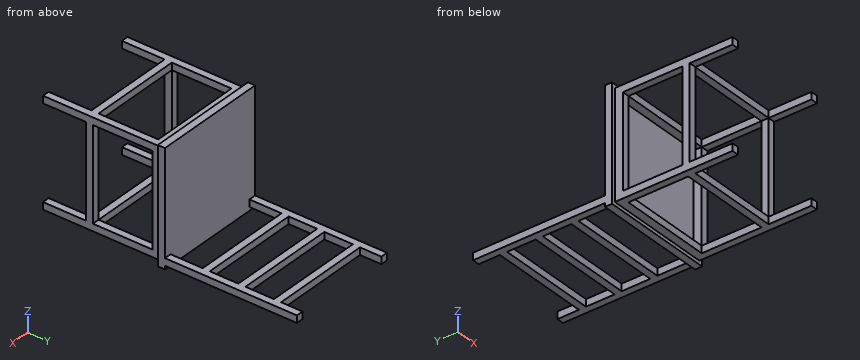
```python
from build123d import *

# Parameters (mm, degrees)
SKETCH1_W            = 406.4
SKETCH1_H            = 406.4
BOSS_EXTRUDE1_DEPTH  = 25.4
SKETCH2_W            = 25.4
SKETCH2_H            = 25.4
SKETCH2_W_2          = 330.2
SKETCH2_H_2          = 330.2
BOSS_EXTRUDE4_DEPTH  = 28.575
SKETCH4_W            = 25.4
SKETCH4_H            = 25.4
BOSS_EXTRUDE5_DEPTH  = 390.525
SKETCH6_W            = 25.4
SKETCH6_H            = 25.4
BOSS_EXTRUDE6_DEPTH  = 355.6
SKETCH8_W            = 25.4
SKETCH8_H            = 25.4
BOSS_EXTRUDE7_DEPTH  = 355.6
SKETCH9_W            = 25.4
SKETCH9_H            = 25.4
BOSS_EXTRUDE8_DEPTH  = 355.6
SKETCH10_W           = 25.4
SKETCH10_H           = 25.4
BOSS_EXTRUDE9_DEPTH  = 355.6
SKETCH11_W           = 25.4
SKETCH11_H           = 25.4
BOSS_EXTRUDE11_DEPTH = 469.9
SKETCH12_W           = 25.4
SKETCH12_H           = 25.4
BOSS_EXTRUDE12_DEPTH = 376.174


with BuildPart() as part:
    # Sketch1 → Boss-Extrude1 (new body)
    with BuildSketch(Plane(origin=(0, 0, 0), x_dir=(1, 0, 0), z_dir=(0, 1, 0))):
        with Locations((203.2, 203.2)):
            Rectangle(SKETCH1_W, SKETCH1_H)
    extrude(amount=BOSS_EXTRUDE1_DEPTH)

    # Sketch2 → Boss-Extrude4 (add)
    with BuildSketch(Plane.XZ):
        with Locations((25.4, -25.4)):
            Rectangle(SKETCH2_W, SKETCH2_H)
        with Locations((203.2, -25.4)):
            Rectangle(SKETCH2_W_2, SKETCH2_H)
        with Locations((25.4, -203.2)):
            Rectangle(SKETCH2_W, SKETCH2_H_2)
        with Locations((203.2, -381)):
            Rectangle(SKETCH2_W_2, SKETCH2_H)
        with Locations((25.4, -381)):
            Rectangle(SKETCH2_W, SKETCH2_H)
        with Locations((381, -381)):
            Rectangle(SKETCH2_W, SKETCH2_H)
        with Locations((381, -203.2)):
            Rectangle(SKETCH2_W, SKETCH2_H_2)
        with Locations((381, -25.4)):
            Rectangle(SKETCH2_W, SKETCH2_H)
    extrude(amount=BOSS_EXTRUDE4_DEPTH)

    # Sketch4 → Boss-Extrude5 (add)
    with BuildSketch(Plane.XZ.offset(28.575)):
        with Locations((25.4, -25.4)):
            Rectangle(SKETCH4_W, SKETCH4_H)
        with Locations((381, -25.4)):
            Rectangle(SKETCH4_W, SKETCH4_H)
        with Locations((381, -381)):
            Rectangle(SKETCH4_W, SKETCH4_H)
        with Locations((25.4, -381)):
            Rectangle(SKETCH4_W, SKETCH4_H)
    extrude(amount=BOSS_EXTRUDE5_DEPTH)

    # Sketch6 → Boss-Extrude6 (add)
    with BuildSketch(Plane(origin=(38.1, 0, 0), x_dir=(0, 0, -1), z_dir=(1, 0, 0))):
        with Locations((25.4, -254)):
            Rectangle(SKETCH6_W, SKETCH6_H)
    extrude(amount=BOSS_EXTRUDE6_DEPTH)

    # Sketch8 → Boss-Extrude7 (add)
    with BuildSketch(Plane(origin=(0, 0, -38.1), x_dir=(-1, 0, 0), z_dir=(0, 0, -1))):
        with Locations((-381, -254)):
            Rectangle(SKETCH8_W, SKETCH8_H)
    extrude(amount=BOSS_EXTRUDE7_DEPTH)

    # Sketch9 → Boss-Extrude8 (add)
    with BuildSketch(Plane.ZY.offset(-368.3)):
        with Locations((-381, -254)):
            Rectangle(SKETCH9_W, SKETCH9_H)
    extrude(amount=BOSS_EXTRUDE8_DEPTH)

    # Sketch10 → Boss-Extrude9 (add)
    with BuildSketch(Plane.XY.offset(-368.3)):
        with Locations((25.4, -254)):
            Rectangle(SKETCH10_W, SKETCH10_H)
    extrude(amount=BOSS_EXTRUDE9_DEPTH)

    # Sketch11 → Boss-Extrude11 (add)
    with BuildSketch(Plane(origin=(0, 25.4, 0), x_dir=(1, 0, 0), z_dir=(0, 1, 0))):
        with Locations((12.7, 381)):
            Rectangle(SKETCH11_W, SKETCH11_H)
        with Locations((393.7, 381)):
            Rectangle(SKETCH11_W, SKETCH11_H)
    extrude(amount=BOSS_EXTRUDE11_DEPTH)

    # Sketch12 → Boss-Extrude12 (add)
    with BuildSketch(Plane.ZY.offset(-381)):
        with Locations((-381, 406.4)):
            Rectangle(SKETCH12_W, SKETCH12_H)
        with Locations((-381, 279.4)):
            Rectangle(SKETCH12_W, SKETCH12_H)
        with Locations((-381, 152.4)):
            Rectangle(SKETCH12_W, SKETCH12_H)
    extrude(amount=BOSS_EXTRUDE12_DEPTH)


solid = part.part
```
Check sheet for the modelled part. Datum: model origin and axes. Units: mm. Give positions to 0.01 mm unless a question says otherwise; leave off trailing zeros. Loops run counter-clockwise (first coordinate to the right, second up) from the corner with the lowest first, then second, coordinate; pieces in that order, holes last. Notation, with made-up numbers: M 10.25,88 L 18.25,88 A17 cw 18.25,94 Z; hole C 0,-23.75 d1. An arc over 180 degrees is marked long. Answer in a Markdown table with one row per item.
1) Cross-section at A-A (x = 265). Count the separate pieces of the cut face and the enclosed holes in it, plus the area to 3 significant figures.
Solutions:
| item | result |
|---|---|
| separate pieces | 6 |
| enclosed holes | 0 |
| area | 15,000 mm^2 |
2) Cross-section at C-C (y = 329). Enter the section's corners in (x, z), plus the area to 3 significant figures.
Solutions:
| item | result |
|---|---|
| outline | M 0,-393.7 L 25.4,-393.7 L 25.4,-368.3 L 0,-368.3 Z; M 381,-393.7 L 406.4,-393.7 L 406.4,-368.3 L 381,-368.3 Z |
| area | 1,290 mm^2 |
3) Thickness scan on line 1 (X direction, y = -252, z = -318); line 2 (Z direction, x = 363.5, y = -1.5); line 3 (Y direction, x = 204, z = -21.5) (3 decimals). Record the ranges inside material, lowest first.
Solutions:
| item | result |
|---|---|
| line 1 | x = 12.7 to 38.1, 368.3 to 393.7 |
| line 2 | z = -393.7 to -368.3, -38.1 to -12.7 |
| line 3 | y = -266.7 to -241.3, -28.575 to 25.4 |
4) Cross-section at B-B (z = -61.5). Enter the section's corners in (x, y) (3 decimals).
Solutions:
| item | result |
|---|---|
| outline | M 0,0 L 12.7,0 L 12.7,-28.575 L 38.1,-28.575 L 38.1,0 L 368.3,0 L 368.3,-28.575 L 393.7,-28.575 L 393.7,0 L 406.4,0 L 406.4,25.4 L 0,25.4 Z; M 12.7,-266.7 L 38.1,-266.7 L 38.1,-241.3 L 12.7,-241.3 Z; M 368.3,-266.7 L 393.7,-266.7 L 393.7,-241.3 L 368.3,-241.3 Z |
5) Cross-section at D-D (y = -109). Enter the section's corners in (x, z).
Solutions:
| item | result |
|---|---|
| outline | M 12.7,-393.7 L 38.1,-393.7 L 38.1,-368.3 L 12.7,-368.3 Z; M 12.7,-38.1 L 38.1,-38.1 L 38.1,-12.7 L 12.7,-12.7 Z; M 368.3,-393.7 L 393.7,-393.7 L 393.7,-368.3 L 368.3,-368.3 Z; M 368.3,-38.1 L 393.7,-38.1 L 393.7,-12.7 L 368.3,-12.7 Z |
6) Depth check by flat-ended pin: pin 1 (12 mm diameter, centred on x = 259, z = -276, fed in from +Y); pin 2 (20.5 mm diameter, centred on y = -135, z = -382.5, fed in from +X); pin 3 (8.5 mm diameter, centred on y = -18.5, z = -236, fed in from -X). Enter the tip coordinate at first touch or a pass-through.
Solutions:
| item | result |
|---|---|
| pin 1 | stops at y = 25.4 |
| pin 2 | stops at x = 393.7 |
| pin 3 | stops at x = 12.7 |
